Autodesk Inventor part; units mm, degrees
ref_plane "YZ Plane" through (0, 0, 0) normal (1, 0, 0) x (0, 1, 0)
ref_plane "XZ Plane" through (0, 0, 0) normal (0, 1, 0) x (-1, 0, 0)
ref_plane "XY Plane" through (0, 0, 0) normal (0, 0, 1) x (1, 0, 0)
sketch "Boceto1" plane through (0, 0, 0) normal (0, 1, 0) x (-1, 0, 0)
  arc A0 (-18, 72.808) -> (20, 72.2842) centre (0, 0) ccw
  line L0 (-18, 72.808) -> (-18, 72.2842)
  line L1 (55, 8) -> (40, 8)
  line L2 (40, 8) -> (40, -42)
  line L3 (40, -42) -> (55, -42)
  line L4 (55, -42) -> (55, 8)
  line L5 (-40, 8) -> (-55, 8)
  line L6 (-55, 8) -> (-55, -42)
  line L7 (-55, -42) -> (-40, -42)
  line L8 (-40, -42) -> (-40, 8)
  line L9 (20, 72.2842) -> (12, 72.2842)
  line L10 (12, 72.2842) -> (12, 25.2842)
  line L11 (-18, 72.808) -> (-12, 72.808)
  line L12 (-12, 72.808) -> (-12, 25.2842)
  line L13 (-18, 72.2842) -> (-18, 72.808)
  line L14 (12, 25.2842) -> (-12, 25.2842)
  line L15 (-30.8486, 25.2842) -> (-30.8486, 25)
  dimension "d0" = 150
  dimension "d1" = 18
  dimension "d3" = 15
  dimension "d4" = 50
  dimension "d5" = 15
  dimension "d6" = 50
  dimension "d7" = 40
  dimension "d8" = 40
  dimension "d28" = 24
  dimension "d29" = 12
  dimension "d33" = 8
  dimension "d34" = 8
  dimension "d36" = 47
extrude "Extrusión1" add sketch "Boceto1" along normal blind 2
sketch "Boceto2" plane through (0, 0, 0) normal (0, 1, 0) x (-1, 0, 0)
  line L0 (-74.7999, 67.2842) -> (80.1068, 67.2842)
  line L1 (80.1068, 67.2842) -> (80.1068, 81.1614)
  line L2 (80.1068, 81.1614) -> (-74.7999, 81.1614)
  line L3 (-74.7999, 81.1614) -> (-74.7999, 67.2842)
  line L4 (20, 72.2842) -> (12, 72.2842)
  point P0 (0, 0)
  dimension "d13" = 5
extrude "Extrusión2" cut sketch "Boceto2" along normal blind 2
sketch "Boceto3" plane through (0, 0, 0) normal (0, 1, 0) x (-1, 0, 0)
  circle A0 centre (-70, 0) radius 2
  circle A1 centre (0, -70) radius 2
  circle A2 centre (70, 0) radius 2
  point P0 (0, 0)
  dimension "d14" = 4
  dimension "d15" = 4
  dimension "d16" = 4
  dimension "d17" = 70
  dimension "d18" = 70
  dimension "d19" = 70
extrude "Extrusión3" cut sketch "Boceto3" along normal mid plane 6
sketch "Boceto6" plane through (0, 0, 0) normal (0, 1, 0) x (-1, 0, 0)
  line L0 (-27, 57.2842) -> (-36.2309, 57.2842)
  arc A0 (-43.4373, 54.8927) -> (-36.2309, 57.2842) centre (-40.2309, 57.2842) ccw
  arc A1 (-27, 57.2842) -> (-23, 53.2842) centre (-23, 57.2842) ccw
  circle A2 centre (-23, 57.2842) radius 2
  arc A3 (25, 53.2842) -> (29, 57.2842) centre (25, 57.2842) ccw
  circle A4 centre (25, 57.2842) radius 2
  arc A5 (36.2309, 57.2842) -> (43.4373, 54.8927) centre (40.2309, 57.2842) ccw
  circle A6 centre (40.2309, 57.2842) radius 2
  circle A7 centre (-40.2309, 57.2842) radius 2
  point P0 (0, 0)
  dimension "d22" = 4
  dimension "d23" = 4
  dimension "d24" = 4
  dimension "d25" = 4
extrude "Extrusión4" cut sketch "Boceto6" along normal mid plane 6
properties part number "Tapa" material "Nilón 6/6"
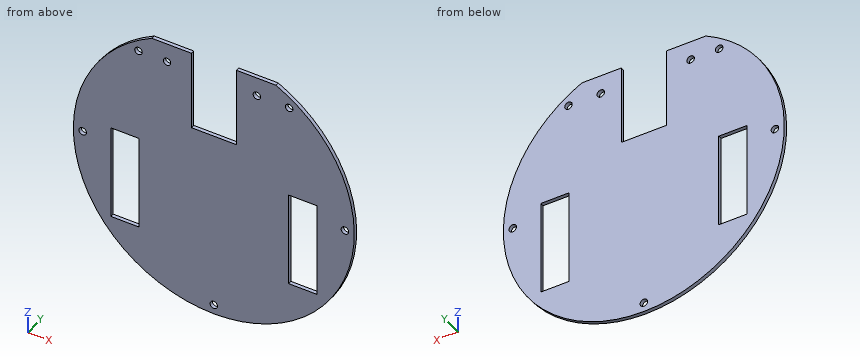
The model under review builds one solid part; all positions refer to its coordinate system, in mm. Coordinates: 2 decimals unless noted, no trailing zeros. Write each loop counter-clockwise with the first axis right and the second up, starting at its lowest first coordinate (ties: lowest second). Pieces come first, ordered by that corner, then holes. Notation, with made-up numbers: (54.5, 15) - (109.5, 15) arc R8 cw to (109.5, 25) - close; hole circle Ø10 at (79, 24.5). An arc over 180 degrees is marked (long way). Answer as a JSON object with one key per item and string values. Group by question number.
1. Add section D-D (x = 31). Give the boundary of the cut face in (y, z).
2. Add section C-C (z = -70). Give the boundary of the cut face in (x, y).
3. To check wall thickness, follow probe 1 along X at (y, z) = (1, 0); probe 2 along X at (y, z) = (1.9, -9.5); probe 3 along X at (y, z) = (0.25, -34). State the ranges of each line that lie inside material, in increasing order.
4. Add section A-A (x = 0). Give the boundary of the cut face in (y, z), plus the area to 3 significant figures.
5. Add section B-B (y = 1.25). Give the number of separate pieces and of enclosed holes in the cut face, plus the area to 3 significant figures.
6. Clearance check with flat-ended pins moving along their axes: pin 1 Ø1 at (x, y) = (45.5, 1) entering from -Z; pin 2 Ø5 at (x, z) = (-70, 0) entering from +Y; pin 3 Ø0.6 at (x, y) = (-46, 0.5) entering from -Z; pin 4 Ø1 at (y, z) = (1, -19.5) entering from -X. State where each tip first meets the part, or that it passes through.
Findings:
{
 "1": {"outline": "(0, -68.29) - (2, -68.29) - (2, 67.28) - (0, 67.28) - close"},
 "2": {"outline": "(-26.93, 0) - (-2, 0) - (-2, 2) - (-26.93, 2) - close; (2, 0) - (26.93, 0) - (26.93, 2) - (2, 2) - close"},
 "3": {"probe 1": "-75 to -72, -68 to -55, -40 to 40, 55 to 68, 72 to 75", "probe 2": "-74.4 to -55, -40 to 40, 55 to 74.4", "probe 3": "-66.85 to -55, -40 to 40, 55 to 66.85"},
 "4": {"outline": "(0, -75) - (2, -75) - (2, -72) - (0, -72) - close; (0, -68) - (2, -68) - (2, 25.28) - (0, 25.28) - close", "area": "193 mm²"},
 "5": {"separate pieces": "1", "enclosed holes": "9", "area": "14,700 mm²"},
 "6": {"pin 1": "z = -60", "pin 2": "y = 2", "pin 3": "z = -59.47", "pin 4": "x = -72.55"}
}
